The listing builds one solid part. Answer for the finished solid, in the listing's coordinates (mm). A direction names the side the tool comes from. Give positions to 0.01 mm unless a question says otherwise; leave off trailing zeros. Write each loop counter-clockwise with the first axis right and the second up, starting at its lowest first coordinate (ties: lowest second). Pieces come first, ordered by that corner, then holes. Notation, with made-up numbers: (48.5, 4) - (82.5, 4) arc R20 cw to (82.5, 11) - close; hole circle Ø7 at (-21.75, 50.25). An arc over 180 degrees is marked (long way). One line per item, written item: value. Start each with the question number.
from build123d import *

# Parameters (mm, degrees)
SKETCH1_W           = 56
SKETCH1_H           = 33
SKETCH1_W_2         = 52
SKETCH1_H_2         = 29
BOSS_EXTRUDE1_DEPTH = 5
SKETCH2_W           = 56
SKETCH2_H           = 33
BOSS_EXTRUDE2_DEPTH = 1
FILLET1_R           = 3
FILLET2_R           = 1
SKETCH3_W           = 8
SKETCH3_H           = 8.4
CUT_EXTRUDE1_DEPTH  = 10
SKETCH9_W           = 3.7
SKETCH9_H           = 2.8
CUT_EXTRUDE4_DEPTH  = 3
BOSS_EXTRUDE6_START = -6
SKETCH5_R           = 4.5
BOSS_EXTRUDE6_DEPTH = 6
SKETCH7_R           = 4.5
SKETCH7_R_2         = 2.5
BOSS_EXTRUDE7_DEPTH = 5
FILLET4_R           = 3
SKETCH8_W           = 20
SKETCH8_H           = 7
CUT_EXTRUDE3_DEPTH  = 3
FILLET5_R           = 1
CHAMFER2_SIZE       = 1
FILLET6_R           = 0.5
SKETCH10_R          = 1
CUT_EXTRUDE5_DEPTH  = 3


with BuildPart() as part:
    # Sketch1 → Boss-Extrude1 (new body)
    with BuildSketch(Plane(origin=(0, 0, 0), x_dir=(1, 0, 0), z_dir=(0, 1, 0))):
        Rectangle(SKETCH1_W, SKETCH1_H)
        Rectangle(SKETCH1_W_2, SKETCH1_H_2, mode=Mode.SUBTRACT)
    extrude(amount=BOSS_EXTRUDE1_DEPTH)

    # Sketch2 → Boss-Extrude2 (add)
    with BuildSketch(Plane.XZ):
        Rectangle(SKETCH2_W, SKETCH2_H)
    extrude(amount=BOSS_EXTRUDE2_DEPTH)

    # Fillet1
    fillet1_edges = [part.edges().sort_by_distance(p)[0] for p in [
        (-28, 2, -16.5),
        (28, 2, -16.5),
        (28, 2, 16.5),
        (-28, 2, 16.5),
    ]]
    fillet(fillet1_edges, radius=FILLET1_R)

    # Fillet2
    fillet2_edges = [part.edges().sort_by_distance(p)[0] for p in [
        (26, 2.5, 14.5),
        (26, 2.5, -14.5),
        (-26, 2.5, -14.5),
        (-26, 2.5, 14.5),
    ]]
    fillet(fillet2_edges, radius=FILLET2_R)

    # Sketch3 → Cut-Extrude1 (cut)
    with BuildSketch(Plane(origin=(28, 0, 0), x_dir=(0, 0, -1), z_dir=(1, 0, 0))):
        with Locations((0, 5)):
            Rectangle(SKETCH3_W, SKETCH3_H)
    extrude(amount=-CUT_EXTRUDE1_DEPTH, mode=Mode.SUBTRACT)

    # Sketch9 → Cut-Extrude4 (cut)
    with BuildSketch(Plane.XY.offset(16.5)):
        with Locations((21.611723176, 5)):
            Rectangle(SKETCH9_W, SKETCH9_H)
    extrude(amount=-CUT_EXTRUDE4_DEPTH, mode=Mode.SUBTRACT)

    # Sketch5 → Boss-Extrude6 (add)
    # profile 1 of 3: a face of its own
    with BuildSketch(Plane.XZ.offset(1).offset(BOSS_EXTRUDE6_START)):
        Polygon((-25, 16.5), (12.5, 16.5), (12.5, 27.55), (-40.5, 27.55), (-40.5, 16.5), (-28, 16.5), align=None)
        with Locations(Location((-34, 21.05, 0), (0, 0, 270))):
            Circle(SKETCH5_R, mode=Mode.SUBTRACT)
        with Locations(Location((6, 21.05, 0), (0, 0, 270))):
            Circle(SKETCH5_R, mode=Mode.SUBTRACT)
    # profile 2 of 3: a face of its own
    with BuildSketch(Plane.XZ.offset(1).offset(BOSS_EXTRUDE6_START)):
        with BuildLine():
            ThreePointArc((-27.252149964, 15.481872988), (-26.2357955, 16.233643993), (-25, 16.5))
            Line((-25, 16.5), (-28, 16.5))
            Line((-28, 16.5), (-28, 15.481872988))
            Line((-28, 15.481872988), (-27.252149964, 15.481872988))
        make_face()
    # profile 3 of 3: a face of its own
    with BuildSketch(Plane.XZ.offset(1).offset(BOSS_EXTRUDE6_START)):
        with BuildLine():
            ThreePointArc((-28, 13.5), (-27.806817583, 14.559138826), (-27.252149964, 15.481872988))
            Line((-27.252149964, 15.481872988), (-28, 15.481872988))
            Line((-28, 15.481872988), (-28, 13.5))
        make_face()
    extrude(amount=BOSS_EXTRUDE6_DEPTH)

    # Sketch7 → Boss-Extrude7 (add)
    # profile 1 of 2: a face of its own
    with BuildSketch(Plane(origin=(0, 5, 0), x_dir=(1, 0, 0), z_dir=(0, 1, 0))):
        with Locations(Location((6, -21.05, 0), (0, 0, 90))):
            Circle(SKETCH7_R)
        with Locations(Location((6, -21.05, 0), (0, 0, 270))):
            Circle(SKETCH7_R_2, mode=Mode.SUBTRACT)
    # profile 2 of 2: a face of its own
    with BuildSketch(Plane(origin=(0, 5, 0), x_dir=(1, 0, 0), z_dir=(0, 1, 0))):
        with Locations(Location((-34, -21.05, 0), (0, 0, 90))):
            Circle(SKETCH7_R)
        with Locations(Location((-34, -21.05, 0), (0, 0, 270))):
            Circle(SKETCH7_R_2, mode=Mode.SUBTRACT)
    extrude(amount=-BOSS_EXTRUDE7_DEPTH)

    # Fillet4
    fillet4_edges = [part.edges().sort_by_distance(p)[0] for p in [
        (-40.5, 2, 16.5),
        (-40.5, 2, 27.55),
        (12.5, 2, 27.55),
        (12.5, 2, 16.5),
        (-28, 2, 16.5),
    ]]
    fillet(fillet4_edges, radius=FILLET4_R)

    # Sketch8 → Cut-Extrude3 (cut)
    with BuildSketch(Plane(origin=(0, 5, 0), x_dir=(1, 0, 0), z_dir=(0, 1, 0))):
        with Locations((-14, -21.05)):
            Rectangle(SKETCH8_W, SKETCH8_H)
    extrude(amount=-CUT_EXTRUDE3_DEPTH, mode=Mode.SUBTRACT)

    # Fillet5
    fillet5_edges = [part.edges().sort_by_distance(p)[0] for p in [
        (-4, 2, 21.05),
        (-4, 3.5, 17.55),
        (-14, 2, 24.55),
        (-4, 3.5, 24.55),
        (-24, 2, 21.05),
        (-24, 3.5, 24.55),
        (-14, 2, 17.55),
        (-24, 3.5, 17.55),
        (-4, 5, 21.05),
        (-14, 5, 17.55),
        (-24, 5, 21.05),
        (-14, 5, 24.55),
    ]]
    fillet(fillet5_edges, radius=FILLET5_R)

    # Chamfer2
    # the kernel refuses this chamfer: 1 mm, written as the material it takes off along each edge
    with BuildSketch(Plane(origin=(12.5, -1, 19.5), x_dir=(0.02749587661058563, 0.9996219169112968, 0), z_dir=(0, 0, 1)), Plane(origin=(-40.5, -1, 24.55), x_dir=(-0.02749587661058908, 0.9996219169112968, 0), z_dir=(0, 0, -1))) as chamfer2_piece_1:
        Polygon((CHAMFER2_SIZE * 0.999621916911, CHAMFER2_SIZE * 0.0274958766106), (-CHAMFER2_SIZE * 0.0274958766106, CHAMFER2_SIZE * 0.999621916911), (0, 0), align=None)
    extrude(amount=5.05, mode=Mode.SUBTRACT)
    with BuildSketch(Plane(origin=(9.5, -1, 27.55), x_dir=(0, 0.9996219169112968, 0.02749587661058563), z_dir=(-1, 0, 0))) as chamfer2_piece_2:
        Polygon((CHAMFER2_SIZE * 0.999621916911, CHAMFER2_SIZE * 0.0274958766106), (-CHAMFER2_SIZE * 0.0274958766106, CHAMFER2_SIZE * 0.999621916911), (0, 0), align=None)
    extrude(amount=47, mode=Mode.SUBTRACT)
    with BuildSketch(Plane(origin=(-31, -1, 16.5), x_dir=(0, 0.9996219169112968, -0.02749587661058563), z_dir=(-1, 0, 0))) as chamfer2_piece_3:
        Polygon((CHAMFER2_SIZE * 0.999621916911, -CHAMFER2_SIZE * 0.0274958766106), (-CHAMFER2_SIZE * 0.0274958766106, -CHAMFER2_SIZE * 0.999621916911), (0, 0), align=None)
    extrude(amount=6.5, mode=Mode.SUBTRACT)
    with BuildSketch(Plane(origin=(-28, -1, -13.5), x_dir=(-0.02749587661058563, 0.9996219169112968, 0), z_dir=(0, 0, 1))) as chamfer2_piece_4:
        Polygon((CHAMFER2_SIZE * 0.999621916911, -CHAMFER2_SIZE * 0.0274958766106), (-CHAMFER2_SIZE * 0.0274958766106, -CHAMFER2_SIZE * 0.999621916911), (0, 0), align=None)
    extrude(amount=27, mode=Mode.SUBTRACT)
    with BuildSketch(Plane(origin=(-37.5, -1, 19.5), x_dir=(-1, 0, 0), z_dir=(0, 0, 1))) as chamfer2_piece_5:
        Polygon((3, -CHAMFER2_SIZE), (3 - CHAMFER2_SIZE, 0), (3, 0), align=None)
    revolve(axis=Axis((-37.5, -1, 19.5), (0, -1, 0)), revolution_arc=90, mode=Mode.SUBTRACT)
    with BuildSketch(Plane(origin=(-37.5, -1, 24.55), x_dir=(0, 0, 1), z_dir=(1, 0, 0))) as chamfer2_piece_6:
        Polygon((3, -CHAMFER2_SIZE), (3 - CHAMFER2_SIZE, 0), (3, 0), align=None)
    revolve(axis=Axis((-37.5, -1, 24.55), (0, -1, 0)), revolution_arc=90, mode=Mode.SUBTRACT)
    with BuildSketch(Plane(origin=(9.5, -1, 24.55), x_dir=(1, 0, 0), z_dir=(0, 0, -1))) as chamfer2_piece_7:
        Polygon((3, -CHAMFER2_SIZE), (3 - CHAMFER2_SIZE, 0), (3, 0), align=None)
    revolve(axis=Axis((9.5, -1, 24.55), (0, -1, 0)), revolution_arc=90, mode=Mode.SUBTRACT)
    with BuildSketch(Plane(origin=(15.5, -1, 19.5), x_dir=(0, 0, -1), z_dir=(1, 0, 0))) as chamfer2_piece_8:
        Polygon((3, CHAMFER2_SIZE), (3 + CHAMFER2_SIZE, 0), (3, 0), align=None)
    revolve(axis=Axis((15.5, -1, 19.5), (0, 1, 0)), revolution_arc=90, mode=Mode.SUBTRACT)
    with BuildSketch(Plane(origin=(-31, -1, 13.5), x_dir=(0, 0, 1), z_dir=(-1, 0, 0))) as chamfer2_piece_9:
        Polygon((3, CHAMFER2_SIZE), (3 + CHAMFER2_SIZE, 0), (3, 0), align=None)
    revolve(axis=Axis((-31, -1, 13.5), (0, 1, 0)), revolution_arc=90, mode=Mode.SUBTRACT)
    with BuildSketch(Plane(origin=(28, -1, -13.5), x_dir=(0.02749587661058563, 0.9996219169112968, 0), z_dir=(0, 0, 1))) as chamfer2_piece_10:
        Polygon((CHAMFER2_SIZE * 0.999621916911, CHAMFER2_SIZE * 0.0274958766106), (-CHAMFER2_SIZE * 0.0274958766106, CHAMFER2_SIZE * 0.999621916911), (0, 0), align=None)
    extrude(amount=27, mode=Mode.SUBTRACT)
    with BuildSketch(Plane(origin=(25, -1, 16.5), x_dir=(0, 0.9996219169112968, 0.02749587661058563), z_dir=(-1, 0, 0))) as chamfer2_piece_11:
        Polygon((CHAMFER2_SIZE * 0.999621916911, CHAMFER2_SIZE * 0.0274958766106), (-CHAMFER2_SIZE * 0.0274958766106, CHAMFER2_SIZE * 0.999621916911), (0, 0), align=None)
    extrude(amount=9.5, mode=Mode.SUBTRACT)
    with BuildSketch(Plane(origin=(-25, -1, -16.5), x_dir=(0, 0.9996219169112968, -0.02749587661058563), z_dir=(1, 0, 0))) as chamfer2_piece_12:
        Polygon((CHAMFER2_SIZE * 0.999621916911, CHAMFER2_SIZE * 0.0274958766106), (-CHAMFER2_SIZE * 0.0274958766106, CHAMFER2_SIZE * 0.999621916911), (0, 0), align=None)
    extrude(amount=50, mode=Mode.SUBTRACT)
    with BuildSketch(Plane(origin=(-25, -1, -13.5), x_dir=(0, 0, -1), z_dir=(1, 0, 0))) as chamfer2_piece_13:
        Polygon((3, CHAMFER2_SIZE), (3 - CHAMFER2_SIZE, 0), (3, 0), align=None)
    revolve(axis=Axis((-25, -1, -13.5), (0, 1, 0)), revolution_arc=90, mode=Mode.SUBTRACT)
    with BuildSketch(Plane(origin=(25, -1, -13.5), x_dir=(0, 0, -1), z_dir=(-1, 0, 0))) as chamfer2_piece_14:
        Polygon((3, -CHAMFER2_SIZE), (3 - CHAMFER2_SIZE, 0), (3, 0), align=None)
    revolve(axis=Axis((25, -1, -13.5), (0, -1, 0)), revolution_arc=90, mode=Mode.SUBTRACT)
    with BuildSketch(Plane(origin=(25, -1, 13.5), x_dir=(0, 0, 1), z_dir=(-1, 0, 0))) as chamfer2_piece_15:
        Polygon((3 - CHAMFER2_SIZE, 0), (3, CHAMFER2_SIZE), (3, 0), align=None)
    revolve(axis=Axis((25, -1, 13.5), (0, 1, 0)), revolution_arc=90, mode=Mode.SUBTRACT)

    # Fillet6
    fillet6_edges = [part.edges().sort_by_distance(p)[0] for p in [
        (27, 0.8, -4),
        (19.761723176, 3.6, 15.5),
        (23.461723176, 3.6, 15.5),
        (27, 0.8, 4),
    ]]
    fillet(fillet6_edges, radius=FILLET6_R)

    # Sketch10 → Cut-Extrude5 (cut)
    with BuildSketch(Plane(origin=(0, 0, 0), x_dir=(1, 0, 0), z_dir=(0, 1, 0))):
        with Locations(Location((4.4, 4.9, 0), (0, 0, 270))):
            Circle(SKETCH10_R)
        with Locations(Location((4.4, -4.3, 0), (0, 0, 270))):
            Circle(SKETCH10_R)
    extrude(amount=-CUT_EXTRUDE5_DEPTH, mode=Mode.SUBTRACT)


solid = part.part
Item 1: Find section A-A on x = -34. Determine the outline of the cut face in (y, z).
Item 2: Find section C-C on x = -18.5. Determine the outline of the cut face in (y, z), plus the area to 3 significant figures.
Item 3: For faces 5 (the flat face through (8, 0, 19)), 6 (the flat face through (20, 3, 16.5)), 7 (the flat face through (-9, 5, 15)), 8 (the flat face through (27, 3, -4)), 9 (the flat face through (26, 0.2, 0.2)), determine the directions among +Z, -Z, +X, -X, +Y, -Y from which every point of the face is accessible in a straight line to the end or side of a thin tool.
Item 4: The mould has two halves that part along Z. Classify faces 1 (the cylindrical face through (8.11, 2.54, 22.39)), 2 (the flat face through (0, 0, 0)), 3 (the conical face through (-39.166, -0.618, 26.253)), 4 (the flat face through (12.5, 3, 22)): +Z half, -Z half, draft (parallel to the pull), parting line (faces both ways), or undercut.
Item 5: Find section D-D on z = 7. Determine the outline of the cut face in (x, y), plus the area to 3 significant figures.
Item 6: Find section B-B on z = 21.05. Give the number of separate pieces and of enclosed holes in the cut face, plus the area to 3 significant figures.
Item 7: Straight lines are drawn through the part: line 1 along Z through (x, y) = (-11, 3.5); line 2 along X through (y, z) = (4.05, 21.05). For each, find the intervals that lie inside material, in ascending order.
Item 8: Each of these flat-tipped pins is pushed along its axis until it touches: pin 1 Ø7 at (x, z) = (-35.5, 22) entering from -Y; pin 2 Ø6 at (x, z) = (6, 21.05) entering from -Y; pin 3 Ø0.6 at (x, z) = (22, 15.5) entering from +Y; pin 4 Ø8.5 at (x, z) = (-8, 3.5) entering from +Y. Where does it stop, or does it pass through?
Values:
1. outline: (-1, 25.55) - (0, 25.55) - (0, 23.55) - (5, 23.55) - (5, 27.55) - (0, 27.55) - (-1, 26.55) - close; (-0.05, 16.55) - (0, 16.5) - (5, 16.5) - (5, 18.55) - (0, 18.55) - (0, 16.55) - close
2. outline: (-1, -15.5) - (0, -16.5) - (5, -16.5) - (5, -14.5) - (0, -14.5) - (0, 14.5) - (5, 14.5) - (5, 16.55) arc R1 ccw to (4, 17.55) - (3, 17.55) arc R1 cw to (2, 18.55) - (2, 23.55) arc R1 cw to (3, 24.55) - (4, 24.55) arc R1 ccw to (5, 25.55) - (5, 27.55) - (0, 27.55) - (-1, 26.55) - close
2. area: 97.3 mm^2
3. face 5: -Y
3. face 6: +Z, +X, +Y, -Y
3. face 7: +Z, -Z, +X, -X, +Y
3. face 8: +X, +Y
3. face 9: +Y
4. face 1: undercut
4. face 2: undercut
4. face 3: +Z half
4. face 4: draft
5. outline: (-28, 0) - (-27, -1) - (27, -1) - (28, 0) - (28, 5) - (26, 5) - (26, 0) - (-26, 0) - (-26, 5) - (-28, 5) - close
5. area: 75.0 mm^2
6. separate pieces: 3
6. enclosed holes: 0
6. area: 189 mm^2
7. line 1: -16.5 to -14.5, 14.5 to 17.55, 24.55 to 27.55
7. line 2: -40.5 to -36.5, -31.5 to -24, -4 to 3.5, 8.5 to 12.5
8. pin 1: y = -1
8. pin 2: y = 0
8. pin 3: y = 3.6
8. pin 4: y = 0
